from build123d import *

# Parameters (mm, degrees)
CROQUIS1_W              = 15
CROQUIS1_H              = 200
SALIENTE_EXTRUIR1_DEPTH = 7
CORTAR_EXTRUIR1_DEPTH   = 201.593371852


with BuildPart() as part:
    # Croquis1 → Saliente-Extruir1 (new body)
    with BuildSketch(Plane(origin=(0, 0, 0), x_dir=(0, 0, -1), z_dir=(1, 0, 0))):
        with Locations((-6.236842105, -71.973684211)):
            Rectangle(CROQUIS1_W, CROQUIS1_H)
    extrude(amount=SALIENTE_EXTRUIR1_DEPTH)

    # Croquis2 → Cortar-Extruir1 (cut, through all)
    with BuildSketch(Plane(origin=(0, 28.026315789, 0), x_dir=(1, 0, 0), z_dir=(0, 1, 0))):
        Polygon((7, -0.736842105), (4, -0.736842105), (4, 0.263157895), (2, 0.263157895), (2, -12.736842105), (4, -12.736842105), (4, -11.736842105), (7, -11.736842105), align=None)
    extrude(amount=-CORTAR_EXTRUIR1_DEPTH, mode=Mode.SUBTRACT)


solid = part.part
The listing builds one solid part. Answer for the finished solid, in the listing's coordinates (mm). Coordinates: 2 decimals unless noted, no trailing zeros. Loops run counter-clockwise (first coordinate to the right, second up) from the corner with the lowest first, then second, coordinate; pieces in that order, holes last.
1) Find section B-B on y = -117.5. Write down the section's boundary in (x, z).
2) Flat-ended cylindrical pins translate along their axes: pin 1 Ø4 at (x, z) = (5.5, 4) entering from -Y; pin 2 Ø4 at (y, z) = (-79, 4) entering from +X. Find the tip coordinate at first contact, or state that the pin passes through.
3) Find section A-A on x = 5.5. Write down the section's boundary in (y, z).
4) Find the intervals of material crossed by L1, parallel to Z at x = 6, y = -43; L2, parallel to X at y = 1.5, z = 0.5; L3, parallel to Z at x = 3.5, y = -157.5, in increasing order.
5) Find section C-C on z = 4. Write down the section's boundary in (x, y), then the cut area to 3 significant figures.
Values:
1. outline: (0, -1.26) - (7, -1.26) - (7, 0.74) - (4, 0.74) - (4, -0.26) - (2, -0.26) - (2, 12.74) - (4, 12.74) - (4, 11.74) - (7, 11.74) - (7, 13.74) - (0, 13.74) - close
2. pin 1: passes through
2. pin 2: stops at x = 2
3. outline: (-171.97, -1.26) - (28.03, -1.26) - (28.03, 0.74) - (-171.97, 0.74) - close; (-171.97, 11.74) - (28.03, 11.74) - (28.03, 13.74) - (-171.97, 13.74) - close
4. L1: z = -1.26 to 0.74, 11.74 to 13.74
4. L2: x = 0 to 2, 4 to 7
4. L3: z = -1.26 to -0.26, 12.74 to 13.74
5. outline: (0, -171.97) - (2, -171.97) - (2, 28.03) - (0, 28.03) - close
5. area: 400 mm2
